For this review, take the finished solid that the model builds, in its own axes (mm). A direction names the side the tool comes from. Give positions to 0.01 mm unless a question says otherwise; leave off trailing zeros. Order: outer loops, then holes, each group sorted by start corner. A loop starts at its lowest first (then second) coordinate and runs counter-clockwise, first axis right, second up. Notation, with made-up numbers: (-8.5, 84.25) -> (30.5, 84.25) arc R21 ccw to (30.5, 91.25) -> close; hole circle Ø3 at (19, 26.25). An arc over 180 degrees is marked (long way). Return JSON: item names as keys, results as strings. Group by question number.
1) For faces 4 (the face through (0, -2, 4)), 5 (the face through (2, -2, 0)), 6 (the face through (-2.06, 0.65, 1.48)), 7 (the face through (-0.756, 0.099, 4.119)), 8 (the face through (2.93, -0.179, 0.955)), list the 3-axis set-ups (+Z, -Z, +X, -X, +Y, -Y) from which the entire face can be reached by the end or side of a thin tool; tool diameter is ignored.
2) Add section B-B (y = 0). Give the boundary of the cut face in (x, z), then the cut area to 3 significant figures.
3) Add section D-D (y = -2). Give the boundary of the cut face in (x, z).
4) Add section A-A (x = 0). Give the boundary of the cut face in (y, z).
5) Add section C-C (z = 3.5). Give the boundary of the cut face in (x, y).
6) To check wall thickness, follow line 1 along Y through (x, z) = (0, 1.8); line 2 along Y through (x, z) = (0, 5.85); line 3 along Z through (x, y) = (-2.25, -3). State the ranges of each line that lie inside material, in increasing order.
7) The part is to be moulded in two halves that separate along X. For faces 1 (the face through (0, -1, 3)), 2 (the face through (1, -1, 6.54)), 3 (the face through (-0.21, -1.61, 5.25)), say which applies: released by +X, released by -X, zero draft, split by the parting line, or undercut.
8) Insertion check: P1, Ø1.5, axis at x = -2.5, z = 1.5, coming from the -Y side; P2, Ø1, axis at x = 0.5, y = -1, coming from the -Z side; P3, Ø1.2, axis at x = 0, y = 0, coming from the -Z side; P4, Ø2, axis at x = 2.5, y = -2.5, coming from the +Z side. Each pin has a flat end and moves straight along its axis. Give the tip position at first contact, or say it passes through.
Autodesk Inventor part; units mm, degrees
ref_plane "XZ Plane" through (0, 0, 0) normal (0, 1, 0) x (-1, 0, 0)
ref_plane "XY Plane" through (0, 0, 0) normal (0, 0, 1) x (1, 0, 0)
sketch "Sketch1" plane through (0, 0, 0) normal (0, 0, 1) x (1, 0, 0)
  circle A0 centre (0, 0) radius 3.81
  dimension "d0" = 7.62
extrude "Extrusion1" add sketch "Sketch1" along normal blind 4
sketch "Sketch2" plane through (0, 0, 4) normal (0, 0, 1) x (1, 0, 0)
  circle A0 centre (0, 0) radius 3.81
  circle A1 centre (0, 0) radius 1.6256
  dimension "d3" = 3.2512
extrude "Extrusion2" add sketch "Sketch2" along normal blind 2.54 contours A1
sketch "Sketch3" plane through (0, 0, 6.54) normal (0, 0, 1) x (1, 0, 0)
  circle A0 centre (0, 0) radius 1.6256
hole "Hole1" at (0, 0, 6.54) direction (0, 0, -1) diameter 1.524 end through all
sketch "Sketch4" plane through (0, 0, 0) normal (0, 0, -1) x (-1, 0, 0)
  circle A0 centre (0, 0) radius 0.762
  circle A1 centre (0, 0) radius 3.81
  circle A2 centre (0, 0) radius 2.159
  dimension "d15" = 4.318
extrude "Extrusion3" cut sketch "Sketch4" against normal blind 3 contours A2
ref_plane "Work Plane1" through (3.81, 0, 0) normal (1, 0, 0) x (0, 1, 0)
sketch "Sketch5" plane through (3.81, 0, 0) normal (1, 0, 0) x (0, 1, 0)
  line L0 (-3.81, 4) -> (3.81, 4)
  line L1 (-3.81, 0) -> (3.81, 0)
  line L2 (0, -1.2) -> (0, 7.2)
  line L3 (-2.159, 3) -> (2.159, 3)
  point P0 (0, 0)
  point P1 (0, 1.524)
  dimension "d16" = 3
  dimension "d17" = 1.524
hole "Hole2" at (3.81, 0, 1.524) direction (-1, 0, 0) diameter 1.1938 end up to surface
sketch "Sketch6" plane through (0, 0, 6.54) normal (0, 0, 1) x (1, 0, 0)
  circle A0 centre (0, 0) radius 0.762
  circle A1 centre (0, 0) radius 1.6256
  circle A2 centre (0, 0) radius 1.2446
  dimension "d25" = 2.4892
extrude "Extrusion4" cut sketch "Sketch6" against normal blind 1.27 contours A2
properties part number "bottom_cap"
Evaluation:
{
 "1": {"face 4": "+Z", "face 5": "-Z, +X, -X, +Y, -Y", "face 6": "-Z", "face 7": "+Z, -Z", "face 8": "+X"},
 "2": {"outline": "(-3.81, 0) -> (-2.16, 0) -> (-2.16, 3) -> (-0.76, 3) -> (-0.76, 5.27) -> (-1.24, 5.27) -> (-1.24, 6.54) -> (-1.63, 6.54) -> (-1.63, 4) -> (-3.81, 4) -> close; (0.76, 3) -> (2.16, 3) -> (2.16, 2.12) -> (3.81, 2.12) -> (3.81, 4) -> (1.63, 4) -> (1.63, 6.54) -> (1.24, 6.54) -> (1.24, 5.27) -> (0.76, 5.27) -> close; (2.16, 0) -> (3.81, 0) -> (3.81, 0.93) -> (2.16, 0.93) -> close", "area": "17.2 mm^2"},
 "3": {"outline": "(-3.24, 0) -> (-0.81, 0) -> (-0.81, 3) -> (0.81, 3) -> (0.81, 0) -> (3.24, 0) -> (3.24, 4) -> (-3.24, 4) -> close"},
 "4": {"outline": "(-3.81, 0) -> (-2.16, 0) -> (-2.16, 3) -> (-0.76, 3) -> (-0.76, 5.27) -> (-1.24, 5.27) -> (-1.24, 6.54) -> (-1.63, 6.54) -> (-1.63, 4) -> (-3.81, 4) -> close; (0.76, 3) -> (2.16, 3) -> (2.16, 0) -> (3.81, 0) -> (3.81, 4) -> (1.63, 4) -> (1.63, 6.54) -> (1.24, 6.54) -> (1.24, 5.27) -> (0.76, 5.27) -> close"},
 "5": {"outline": "circle Ø7.62 at (0, 0); hole circle Ø1.52 at (0, 0)"},
 "6": {"line 1": "-3.81 to -2.16, 2.16 to 3.81", "line 2": "-1.63 to -1.24, 1.24 to 1.63", "line 3": "0 to 4"},
 "7": {"face 1": "undercut", "face 2": "zero draft", "face 3": "split by the parting line"},
 "8": {"P1": "y = -3.38", "P2": "z = 3", "P3": "through", "P4": "z = 4"}
}
